Drawing for the job (mm, zero at the part's lowest x, y, z). A direction names the side the tool comes from. Coordinates: 2 decimals unless noted, no trailing zeros. Loops run counter-clockwise (first coordinate to the right, second up) from the corner with the lowest first, then second, coordinate; pieces in that order, holes last. Notation, with made-up numbers: (83.25, -27.75) -> (135.25, -27.75) arc R24 cw to (135.25, -4.75) -> close; hole circle Ø3 at (-29, -17.75). An arc over 180 degrees is marked (long way). Write each question's results on one line, items separated by ' | '.
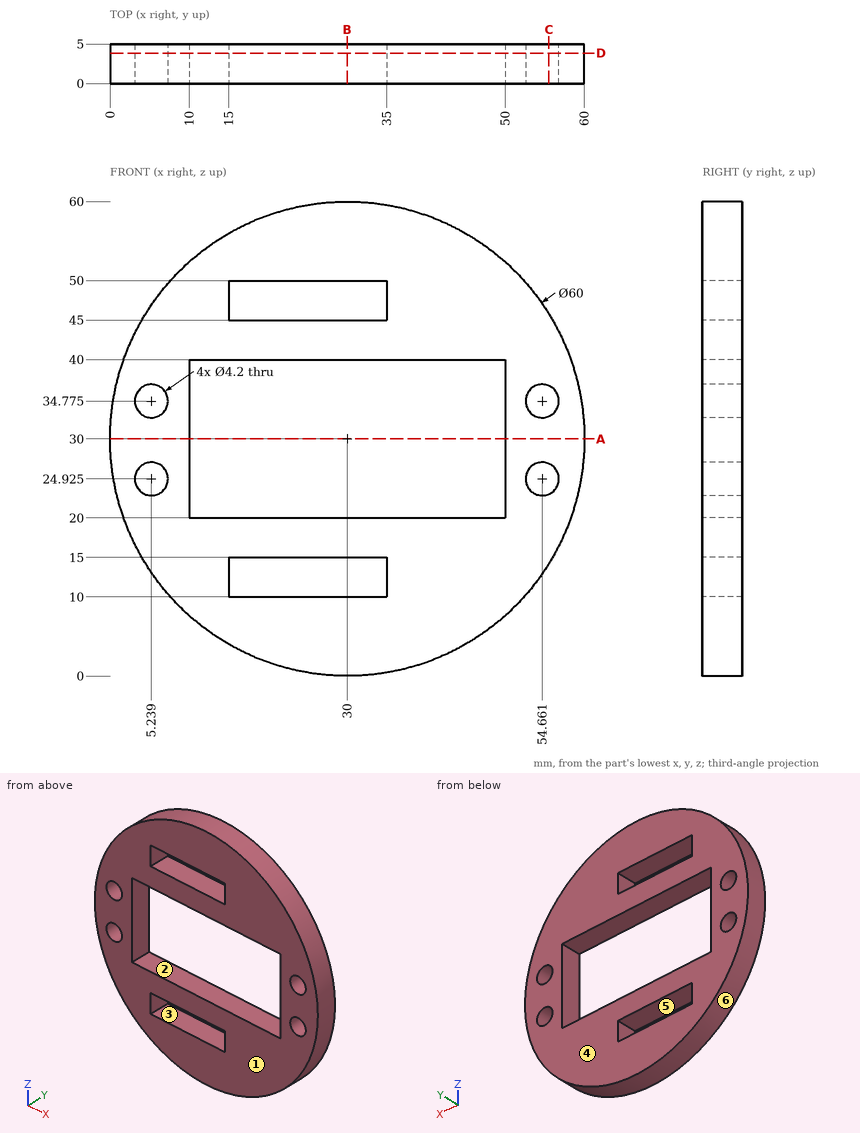
1) Slice it at D-D (y = 3.85). Write the cut outline in (x, z) (3 decimals).
Outcome:
outline: circle Ø60 at (30, 30); hole circle Ø4.2 at (5.239, 24.925); hole circle Ø4.2 at (5.239, 34.775); hole (10, 20) -> (50, 20) -> (50, 40) -> (10, 40) -> close; hole (15, 10) -> (35, 10) -> (35, 15) -> (15, 15) -> close; hole (15, 45) -> (35, 45) -> (35, 50) -> (15, 50) -> close; hole circle Ø4.2 at (54.661, 24.925); hole circle Ø4.2 at (54.661, 34.775)
2) Which spindle directions (+Z, -Z, +X, -X, +Y, -Y) get a long thin tool onto all of the face, cutting with end or side? Do the marked faces 1 and 2. Say none if no direction does.
Outcome:
face 1: +Z, -Z, +X, -X, -Y | face 2: +Y, -Y
3) Drill centre lines: L1, parallel to Z at x = 30, y = 3; L2, parallel to Z at x = 56.5, y = 0.5; L3, parallel to Z at x = 5.5, y = 4.7. Where is each one in solid material? Low to high. Write a range as from..to.
Outcome:
L1: z = 0..10, 15..20, 40..45, 50..60 | L2: z = 15.94..23.91, 25.94..33.76, 35.79..44.06 | L3: z = 12.69..22.84, 27.01..32.69, 36.86..47.31
4) Slice it at C-C (x = 55.5). Write the cut outline in (y, z).
Outcome:
outline: (0, 14.2) -> (5, 14.2) -> (5, 23) -> (0, 23) -> close; (0, 26.85) -> (5, 26.85) -> (5, 32.85) -> (0, 32.85) -> close; (0, 36.7) -> (5, 36.7) -> (5, 45.8) -> (0, 45.8) -> close
5) Slice it at B-B (x = 30). Write the cut outline in (y, z).
Outcome:
outline: (0, 0) -> (5, 0) -> (5, 10) -> (0, 10) -> close; (0, 15) -> (5, 15) -> (5, 20) -> (0, 20) -> close; (0, 40) -> (5, 40) -> (5, 45) -> (0, 45) -> close; (0, 50) -> (5, 50) -> (5, 60) -> (0, 60) -> close
6) Pin check, flat tips, straight feed: pin 1 (2.5 mm diameter, centred on x = 21.5, y = 2, fed in from -Z); pin 2 (2.5 mm diameter, centred on y = 2.5, z = 13, fed in from -X); pin 3 (1 mm diameter, centred on x = 47, y = 3.5, fed in from +Z) (1 decimal). Stop position of each tip, or through.
Outcome:
pin 1: stops at z = 0.89 | pin 2: stops at x = 4.47 | pin 3: stops at z = 55.1
7) Two-plate mould, pull along Z, no slides. Class the marked faces 3, 4, 5 and 6: pulls with the +Z half, pulls with the -Z half, needs draft (parallel to the pull), parting line crosses it, or undercut.
Outcome:
face 3: undercut | face 4: needs draft | face 5: undercut | face 6: parting line crosses it
8) Slice it at A-A (z = 30). Write the cut outline in (x, y), then the cut area to 3 significant figures.
Outcome:
outline: (0, 0) -> (10, 0) -> (10, 5) -> (0, 5) -> close; (50, 0) -> (60, 0) -> (60, 5) -> (50, 5) -> close | area: 100 mm^2
